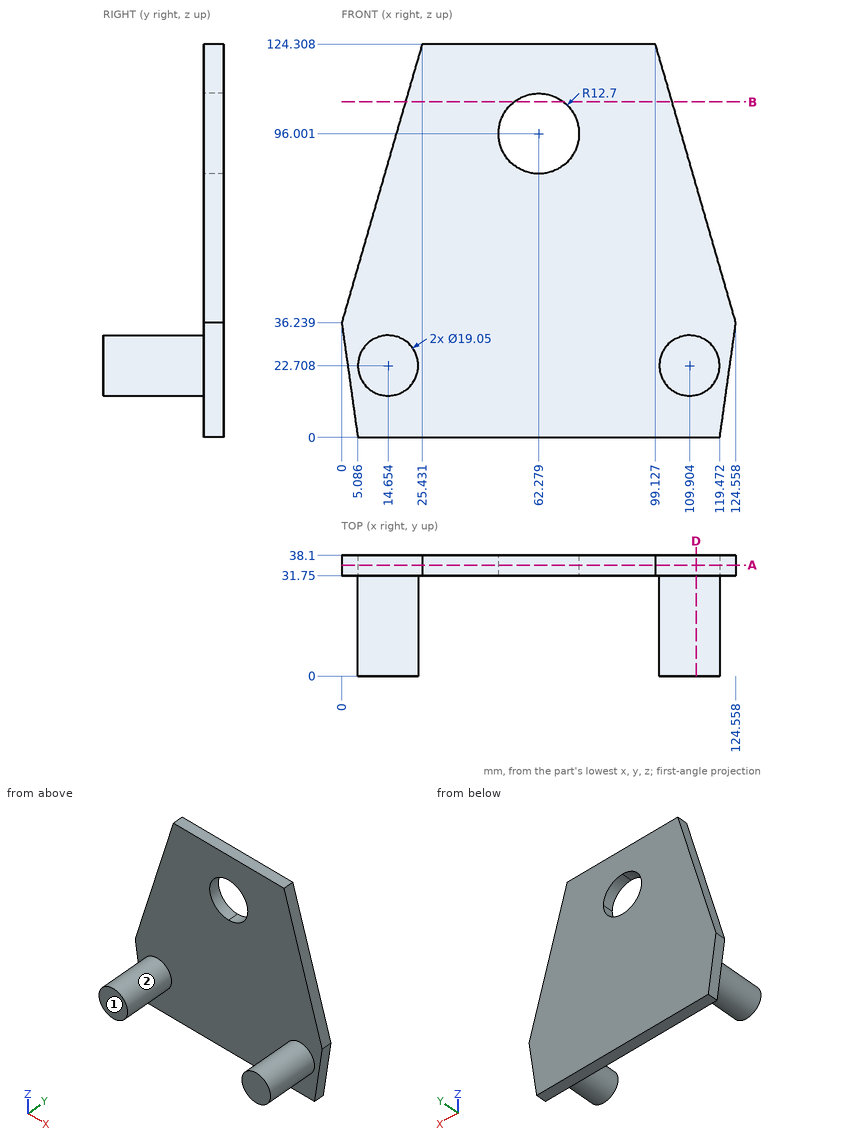
Drawing for the job (mm, zero at the part's lowest x, y, z). A direction names the side the tool comes from. Coordinates: 2 decimals unless noted, no trailing zeros. Order: outer loops, then holes, each group sorted by start corner. A loop starts at its lowest first (then second) coordinate and runs counter-clockwise, first axis right, second up. Notation, with made-up numbers: (40, 51) -> (68, 51) arc R25 ccw to (68, 67) -> close; hole circle Ø7 at (65, 89.25). An arc over 180 degrees is marked (long way). Answer in a Markdown table with one row per item.
1) Flat gauge pins, fed straight in: P1, Ø1, axis at x = 14.5, y = 4, coming from the -Z side; P2, Ø4, axis at y = 33.5, z = 76.5, coming from the +X side; P3, Ø5, axis at y = 13, z = 17, coming from the +X side. Where does each tip first touch, or does it go through?
Check values:
| item | result |
|---|---|
| P1 | z = 13.18 |
| P2 | x = 113.51 |
| P3 | x = 118.87 |
2) Band-saw the part on D-D (x = 112). List the corners of the cut face in (y, z).
Check values:
| item | result |
|---|---|
| outline | (0, 13.42) -> (31.75, 13.42) -> (31.75, 0) -> (38.1, 0) -> (38.1, 79.73) -> (31.75, 79.73) -> (31.75, 32) -> (0, 32) -> close |
3) Band-saw the part on A-A (y = 35). List the corners of the cut face in (x, z).
Check values:
| item | result |
|---|---|
| outline | (0, 36.24) -> (5.09, 0) -> (119.47, 0) -> (124.56, 36.24) -> (99.13, 124.31) -> (25.43, 124.31) -> close; hole circle Ø25.4 at (62.28, 96) |
4) Drill centre lines: line 1 (X direction, y = 14, z = 22.5); line 2 (Y direction, x = 5, z = 17); line 3 (X direction, y = 32, z = 99) (1 decimal). Where is each one in solid material? Low to high.
Check values:
| item | result |
|---|---|
| line 1 | 5.13 to 24.18, 100.38 to 119.43 |
| line 2 | 31.75 to 38.1 |
| line 3 | 18.1 to 49.9, 74.6 to 106.4 |
5) Band-saw the part on B-B (z = 106). List the corners of the cut face in (x, y), and give its area (3 significant figures).
Check values:
| item | result |
|---|---|
| outline | (20.14, 31.75) -> (54.45, 31.75) -> (54.45, 38.1) -> (20.14, 38.1) -> close; (70.11, 31.75) -> (104.41, 31.75) -> (104.41, 38.1) -> (70.11, 38.1) -> close |
| area | 436 mm2 |
6) Which spindle directions (+Z, -Z, +X, -X, +Y, -Y) get a long thin tool onto all of the face, cutting with end or side? Do the marked faces 1 and 2. Say none if no direction does.
Check values:
| item | result |
|---|---|
| face 1 | +Z, -Z, +X, -X, -Y |
| face 2 | -Y |
